from build123d import *

# Parameters (mm, degrees)
FILLET1_R           = 1
SKETCH2_W           = 13.18647025
SKETCH2_H           = 12.34139231
BOSS_EXTRUDE1_DEPTH = 1.6
BOSS_EXTRUDE2_START = -6.5
SKETCH2_2_W         = 13.18647025
SKETCH2_2_H         = 12.34139231
BOSS_EXTRUDE2_DEPTH = 1.6
BOSS_EXTRUDE3_DEPTH = 12.341392


with BuildPart() as part:
    # Sketch1 → Revolve1 (revolve)
    with BuildSketch(Plane.XY):
        Polygon((-3, 5), (-3, 2.5), (-6, 0), (-6, -1), (0, -1), (0, 5), align=None)
    revolve(axis=Axis((0, -1, 0), (0, 1, 0)))

    # Fillet1
    fillet1_edges = [part.edges().sort_by_distance(p)[0] for p in [
        (3, 5, 0),
        (6, 0, 0),
        (3, 2.5, 0),
    ]]
    fillet(fillet1_edges, radius=FILLET1_R)

    # Sketch2 → Boss-Extrude1 (add)
    with BuildSketch(Plane.XZ.offset(1)):
        Rectangle(SKETCH2_W, SKETCH2_H)
    extrude(amount=BOSS_EXTRUDE1_DEPTH)



with BuildPart() as body_2:
    # Sketch2<2> → Boss-Extrude2 (new body)
    with BuildSketch(Plane.XZ.offset(1).offset(BOSS_EXTRUDE2_START)):
        Rectangle(SKETCH2_2_W, SKETCH2_2_H)
    extrude(amount=-BOSS_EXTRUDE2_DEPTH)


with BuildPart() as part_1:
    add(part.part)

    add(body_2.part)  # Boss-Extrude3 merges body 2
    # Sketch4 → Boss-Extrude3 (add)
    with BuildSketch(Plane.XY.offset(6.170696155)):
        with BuildLine():
            Line((6.593235125, 5.5), (21.616366257, 5.5))
            ThreePointArc((21.616366257, 5.5), (24.866366257, 2.25), (21.616366257, -1))
            Line((21.616366257, -1), (6.593235125, -1))
            Line((6.593235125, -1), (6.593235125, -2.6))
            Line((6.593235125, -2.6), (21.616366257, -2.6))
            ThreePointArc((21.616366257, -2.6), (26.466366257, 2.25), (21.616366257, 7.1))
            Line((21.616366257, 7.1), (6.593235125, 7.1))
            Line((6.593235125, 7.1), (6.593235125, 5.5))
        make_face()
    extrude(amount=-BOSS_EXTRUDE3_DEPTH)


solid = part_1.part
Build history of the part. All positions in model axes, mm. A direction names the side the tool comes from. Give positions to 0.01 mm unless a question says otherwise; leave off trailing zeros. Loops run counter-clockwise (first coordinate to the right, second up) from the corner with the lowest first, then second, coordinate; pieces in that order, holes last. Notation, with made-up numbers: (12, 87.5) - (57, 87.5) arc R13 ccw to (57, 110.5) - close; hole circle Ø10 at (77, -39). An arc over 180 degrees is marked (long way). Write item = value, one per line. Start each with the question number.
1) Drop flat-ended pins along their axis: pin 1 Ø5 at (y, z) = (1, -4.5) entering from +X; pin 2 Ø1 at (y, z) = (1, 1) entering from -X. Give the stop position or say it passes through.
2) Pull direction X, two halves, no side cores. Call faces 1 (the flat face through (0, 5, 0)), 2 (the flat face through (-6.593, 6, 0)), 3 (the cylindrical face through (24.866, 2.321, 0.086)): +X half, -X half, draft (parallel to the pull), parting line (faces both ways), or undercut.
3) Probe probe 1 along Y at (x, z) = (21, -0.75); probe 2 along X at (y, z) = (2, -0.75); probe 3 along X at (y, z) = (1.75, 1.5). List the from-to ranges inside material, lowest first. Write a range as from..to.
4) Band-saw the part on B-B on y = -1.5. Give the cut face in (x, z).
5) Band-saw the part on A-A on x = 20. Give the cut face in (y, z), plus the area to 3 significant figures.
6) Tool access for faces 4 (the flat face through (7, 5.5, 0)), 5 (the cylindrical face through (0.78, -0.74, 5.95)), 6 (the cylindrical face through (26.465, 2.143, 0.086)): list every direction of +Z, -Z, +X, -X, +Y, -Y with a clear straight run to the whole face (end or side of a thin tool).
Final values:
q1.pin_1 = 26.47
q1.pin_2 = -5.31
q2.face_1 = draft
q2.face_2 = -X half
q2.face_3 = undercut
q3.probe_1 = -2.6..-1, 5.5..7.1
q3.probe_2 = -3.52..3.52, 24.86..26.46
q3.probe_3 = -3.6..3.6, 24.83..26.44
q4.outline = (-6.59, -6.17) - (24.69, -6.17) - (24.69, 6.17) - (-6.59, 6.17) - close
q5.outline = (-2.6, -6.17) - (-1, -6.17) - (-1, 6.17) - (-2.6, 6.17) - close; (5.5, -6.17) - (7.1, -6.17) - (7.1, 6.17) - (5.5, 6.17) - close
q5.area = 39.5 mm²
q6.face_4 = +Z, -Z, -X
q6.face_5 = none
q6.face_6 = +Z, -Z, +X
